```python
from build123d import *

# Parameters (mm, degrees)
SKETCH4_R                  = 1.651
SKETCH4_R_2                = 1.17475
BOSS_EXTRUDE1_DEPTH        = 1.5875
BOSS_EXTRUDE1_2_DEPTH      = 1.5875
SKETCH5_R                  = 1.14935
BOSS_EXTRUDE2_DEPTH        = 0.762
LPATTERN1_COUNT            = 2
LPATTERN1_PITCH            = 6.35
SKETCH7_R                  = 1.14935
BOSS_EXTRUDE3_DEPTH        = 0.762
SKETCH8_R                  = 1.14935
BOSS_EXTRUDE4_DEPTH        = 3.81
BOSS_EXTRUDE4_DEPTH_BACK   = 3.81
BOSS_EXTRUDE4_2_DEPTH      = 3.81
BOSS_EXTRUDE4_2_DEPTH_BACK = 3.81
LPATTERN2_COUNT            = 2
LPATTERN2_PITCH            = 12.7


with BuildPart() as part:
    # Sketch4 → Boss-Extrude1 (new body, symmetric)
    with BuildSketch(Plane.XY):
        with Locations((-3.175, 0)):
            Circle(SKETCH4_R)
        with Locations((-3.175, 0)):
            Circle(SKETCH4_R_2, mode=Mode.SUBTRACT)
    extrude(amount=BOSS_EXTRUDE1_DEPTH, both=True)


with BuildPart() as body_2:
    # Sketch4 → Boss-Extrude1 2 (new body, symmetric)
    with BuildSketch(Plane.XY):
        with Locations((3.175, 0)):
            Circle(SKETCH4_R)
        with Locations((3.175, 0)):
            Circle(SKETCH4_R_2, mode=Mode.SUBTRACT)
    extrude(amount=BOSS_EXTRUDE1_2_DEPTH, both=True)


with BuildPart() as body_3:
    # Sketch5 → Boss-Extrude2 (new body)
    with BuildSketch(Plane.XY.offset(1.5875)):
        with BuildLine():
            ThreePointArc((-2.342877482, 2.879371452), (-6.1722, 0), (-2.342877482, -2.879371452))
            ThreePointArc((-2.342877482, -2.879371452), (0, -2.54762), (2.342877482, -2.879371452))
            ThreePointArc((2.342877482, -2.879371452), (6.1722, 0), (2.342877482, 2.879371452))
            ThreePointArc((2.342877482, 2.879371452), (0, 2.54762), (-2.342877482, 2.879371452))
        make_face()
        with Locations((-3.175, 0)):
            Circle(SKETCH5_R, mode=Mode.SUBTRACT)
        with Locations((3.175, 0)):
            Circle(SKETCH5_R, mode=Mode.SUBTRACT)
    extrude(amount=BOSS_EXTRUDE2_DEPTH)


with BuildPart() as lpattern1_1:
    # LPattern1: pattern copy
    add(body_2.part.moved(Location(Vector(1, 0, 0) * (1 * LPATTERN1_PITCH))))


with BuildPart() as body_5:
    # Sketch7 → Boss-Extrude3 (new body)
    with BuildSketch(Plane.XY.offset(-2.4003)):
        with BuildLine():
            ThreePointArc((3.931045679, 2.526853989), (0.537464, 0), (3.931045679, -2.526853989))
            ThreePointArc((3.931045679, -2.526853989), (6.35, -2.17272892), (8.768954321, -2.526853989))
            ThreePointArc((8.768954321, -2.526853989), (12.162536, 0), (8.768954321, 2.526853989))
            ThreePointArc((8.768954321, 2.526853989), (6.35, 2.17272892), (3.931045679, 2.526853989))
        make_face()
        with Locations((3.175, 0)):
            Circle(SKETCH7_R, mode=Mode.SUBTRACT)
        with Locations((9.525, 0)):
            Circle(SKETCH7_R, mode=Mode.SUBTRACT)
    extrude(amount=-BOSS_EXTRUDE3_DEPTH)


with BuildPart() as body_6:
    # Mirror1: mirrored copy
    add(body_3.part.mirror(Plane.XY))


with BuildPart() as body_7:
    # Mirror1 2: mirrored copy
    add(body_5.part.mirror(Plane.XY))


with BuildPart() as body_8:
    # Sketch8 → Boss-Extrude4 (new body, two sides)
    with BuildSketch(Plane.XY) as boss_extrude4_sk:
        with Locations((3.175, 0)):
            Circle(SKETCH8_R)
    extrude(amount=BOSS_EXTRUDE4_DEPTH)
    extrude(boss_extrude4_sk.sketch, amount=-BOSS_EXTRUDE4_DEPTH_BACK)


with BuildPart() as body_9:
    # Sketch8 → Boss-Extrude4 2 (new body, two sides)
    with BuildSketch(Plane.XY) as boss_extrude4_2_sk:
        with Locations((9.525, 0)):
            Circle(SKETCH8_R)
    extrude(amount=BOSS_EXTRUDE4_2_DEPTH)
    extrude(boss_extrude4_2_sk.sketch, amount=-BOSS_EXTRUDE4_2_DEPTH_BACK)


with BuildPart() as lpattern2_1:
    # LPattern2: pattern copy
    add(body_9.part.moved(Location(Vector(1, 0, 0) * (1 * LPATTERN2_PITCH))))


with BuildPart() as lpattern2_2:
    # LPattern2: pattern copy
    add(body_8.part.moved(Location(Vector(1, 0, 0) * (1 * LPATTERN2_PITCH))))


with BuildPart() as lpattern2_3:
    # LPattern2: pattern copy
    add(body_7.part.moved(Location(Vector(1, 0, 0) * (1 * LPATTERN2_PITCH))))


with BuildPart() as lpattern2_4:
    # LPattern2: pattern copy
    add(body_6.part.moved(Location(Vector(1, 0, 0) * (1 * LPATTERN2_PITCH))))


with BuildPart() as lpattern2_5:
    # LPattern2: pattern copy
    add(body_5.part.moved(Location(Vector(1, 0, 0) * (1 * LPATTERN2_PITCH))))


with BuildPart() as lpattern2_6:
    # LPattern2: pattern copy
    add(lpattern1_1.part.moved(Location(Vector(1, 0, 0) * (1 * LPATTERN2_PITCH))))


with BuildPart() as lpattern2_7:
    # LPattern2: pattern copy
    add(body_3.part.moved(Location(Vector(1, 0, 0) * (1 * LPATTERN2_PITCH))))


with BuildPart() as lpattern2_8:
    # LPattern2: pattern copy
    add(body_2.part.moved(Location(Vector(1, 0, 0) * (1 * LPATTERN2_PITCH))))


with BuildPart() as lpattern2_9:
    # LPattern2: pattern copy
    add(part.part.moved(Location(Vector(1, 0, 0) * (1 * LPATTERN2_PITCH))))


with BuildPart() as body_2_1:
    add(body_2.part)

    # Combine1: union body 3, LPattern1_1, body 5, body 6, body 7, body 8, body 9, LPattern2_1, LPattern2_2, LPattern2_3, LPattern2_4, LPattern2_5, LPattern2_7, LPattern2_8, LPattern2_9, part
    add(body_3.part)
    add(lpattern1_1.part)
    add(body_5.part)
    add(body_6.part)
    add(body_7.part)
    add(body_8.part)
    add(body_9.part)
    add(lpattern2_1.part)
    add(lpattern2_2.part)
    add(lpattern2_3.part)
    add(lpattern2_4.part)
    add(lpattern2_5.part)
    add(lpattern2_7.part)
    add(lpattern2_8.part)
    add(lpattern2_9.part)
    add(part.part)


solid = body_2_1.part
```
Here's how the part is built. I have some questions about the finished solid (model axes, mm). A direction names the side the tool comes from. Give positions to 0.01 mm unless a question says otherwise; leave off trailing zeros. Order: outer loops, then holes, each group sorted by start corner. A loop starts at its lowest first (then second) coordinate and runs counter-clockwise, first axis right, second up. Notation, with made-up numbers: (56, -9) -> (60, -9) arc R13 cw to (60, -5) -> close; hole circle Ø3 at (17, -33). An arc over 180 degrees is marked (long way). Use CSV: the item, a comma, the result in double quotes. Start each with the question number.
Item 1: Suppose I cut it at D-D (y = 0). Give the number of separate pieces and of enclosed holes in the cut face, and give its area (3 significant figures).
Item 2: On a 3-axis mill with a long thin cutter (end or side, diameter ignored), from which of +Z, -Z, +X, -X, +Y, -Y can I reach the whole of each face in a straight line? I mean faces 4 (the flat face through (19, 0, 3.162)), 5 (the cylindrical face through (8.613, -0.699, -3.482)), 6 (the flat face through (3, 0, -3.81)), 7 (the flat face through (19, 1, 2.4)). Say none if no direction works.
Item 3: Suppose I cut it at B-B (x = 20.5). List the corners of the cut face in (y, z) for me, and give its area (3 significant figures).
Item 4: If I drill on probe 1 along X at (y, z) = (-0.45, -3.25); probe 2 along Z at (x, y) = (0, -1.2); probe 3 along Z at (x, y) = (19, 2.1), over which ranges is the centre line in solid material (lowest first)? Write a range as [from, to].
Item 5: Suppose I cut it at A-A (z = 2). List the corners of the cut face in (x, y) for me (1 decimal), and give its area (3 significant figures).
Item 6: Thinking about a two-plate mould opening in Z: for faces 1 (the flat face through (0, 0, -2.35)), 2 (the flat face through (6, 0, 3.162)), 3 (the cylindrical face through (0.54, 0.07, 2.78)), which applies, pulls with the +Z half, pulls with the -Z half, needs draft (parallel to the pull), parting line crosses it, or undercut?
Item 7: I'm going to push flat-ended pins straight in: P1, Ø4, axis at x = 19, z = 0, coming from the +Y side; P2, Ø1.4, axis at x = -3.175, y = 0, coming from the +Z side; P3, Ø2.5, axis at x = 6, y = -0.5, coming from the -Z side; P4, Ø1, axis at y = 0.5, z = 0, coming from the -X side. Where does each tip first touch, or does it pass through?
Answer block:
1,separate pieces,"2"
1,enclosed holes,"10"
1,area,"127 mm^2"
2,face 4,"+Z"
2,face 5,"-Z"
2,face 6,"-Z, +X, -X, +Y, -Y"
2,face 7,"none"
3,outline,"(-2.3, -3.16) -> (2.3, -3.16) -> (2.3, -2.4) -> (-2.3, -2.4) -> close; (-2.3, 2.4) -> (2.3, 2.4) -> (2.3, 3.16) -> (-2.3, 3.16) -> close"
3,area,"7.01 mm^2"
4,probe 1,"x = [2.12, 4.23], [8.47, 10.58], [14.82, 16.93], [21.17, 23.28]"
4,probe 2,"z = [-2.35, -1.59], [1.59, 2.35]"
4,probe 3,"z = [-3.16, -2.4], [2.4, 3.16]"
5,outline,"(-2.3, -2.9) arc R8.4 cw to (2.3, -2.9) arc R3 ccw (long way) to (2.3, 2.9) arc R8.4 cw to (-2.3, 2.9) arc R3 ccw (long way) to start; (10.4, -2.9) arc R8.4 cw to (15, -2.9) arc R3 ccw (long way) to (15, 2.9) arc R8.4 cw to (10.4, 2.9) arc R3 ccw (long way) to start; circle Ø2.3 at (22.2, 0); hole circle Ø2.3 at (-3.2, 0)"
5,area,"126 mm^2"
6,face 1,"undercut"
6,face 2,"pulls with the +Z half"
6,face 3,"needs draft"
7,P1,"stops at y = 2.31"
7,P2,"passes through"
7,P3,"stops at z = -3.16"
7,P4,"stops at x = -4.83"
